The model under review builds one solid part; all positions refer to its coordinate system, in mm. Face numbers are marked on the shaded views. A direction names the side the tool comes from. Round coordinates to 2 decimals unless told otherwise and drop trailing zeros. Order: outer loops, then holes, each group sorted by start corner. A loop starts at its lowest first (then second) coordinate and runs counter-clockwise, first axis right, second up.
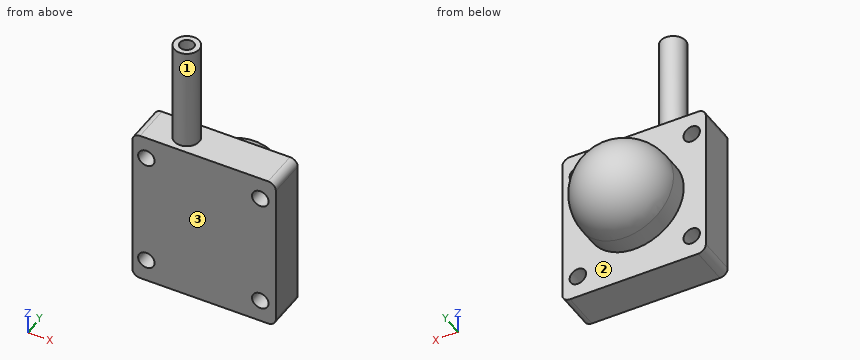
```python
from build123d import *

# Parameters (mm, degrees)
SKETCH1_W           = 27.860395724
SKETCH1_H           = 30.792543072
SKETCH1_R           = 1.6
BOSS_EXTRUDE1_DEPTH = 7.5
SKETCH2_R           = 9.5
BOSS_EXTRUDE2_DEPTH = 3.5
REVOLVE3_ANGLE      = 180
FILLET1_R           = 1.5
SKETCH4_R           = 2.416047387
SKETCH4_R_2         = 1.358434459
BOSS_EXTRUDE3_DEPTH = 20


with BuildPart() as part:
    # Sketch1 → Boss-Extrude1 (new body)
    with BuildSketch(Plane(origin=(0, 0, 0), x_dir=(1, 0, 0), z_dir=(0, 1, 0))):
        with Locations((0.138729437, 0)):
            Rectangle(SKETCH1_W, SKETCH1_H)
        with Locations(Location((-11.05, 11.05, 0), (0, 0, 270))):
            Circle(SKETCH1_R, mode=Mode.SUBTRACT)
        with Locations(Location((11.05, 11.05, 0), (0, 0, 270))):
            Circle(SKETCH1_R, mode=Mode.SUBTRACT)
        with Locations(Location((-11.05, -11.05, 0), (0, 0, 90))):
            Circle(SKETCH1_R, mode=Mode.SUBTRACT)
        with Locations(Location((11.05, -11.05, 0), (0, 0, 90))):
            Circle(SKETCH1_R, mode=Mode.SUBTRACT)
    extrude(amount=BOSS_EXTRUDE1_DEPTH)

    # Sketch2 → Boss-Extrude2 (add)
    with BuildSketch(Plane(origin=(0, 7.5, 0), x_dir=(1, 0, 0), z_dir=(0, 1, 0))):
        with Locations(Location((0, 0, 0), (0, 0, 270))):
            Circle(SKETCH2_R)
    extrude(amount=BOSS_EXTRUDE2_DEPTH)

    # Sketch3 → Revolve3 (revolve)
    with BuildSketch(Plane(origin=(0, 11, 0), x_dir=(1, 0, 0), z_dir=(0, 1, 0))):
        with BuildLine():
            Line((-9.5, 0), (9.5, 0))
            ThreePointArc((9.5, 0), (0, 9.5), (-9.5, 0))
        make_face()
    revolve(axis=Axis((-9.5, 11, 0), (1, 0, 0)), revolution_arc=REVOLVE3_ANGLE)

    # Fillet1
    fillet1_edges = [part.edges().sort_by_distance(p)[0] for p in [
        (-13.791468425, 3.75, -15.396271536),
        (14.068927299, 3.75, -15.396271536),
        (14.068927299, 3.75, 15.396271536),
        (-13.791468425, 3.75, 15.396271536),
    ]]
    fillet(fillet1_edges, radius=FILLET1_R)

    # Sketch4 → Boss-Extrude3 (add)
    with BuildSketch(Plane.XY.offset(15.396271536)):
        with Locations(Location((-5.220214875, 3.559374136, 0), (0, 0, 180))):
            Circle(SKETCH4_R)
        with Locations((-5.220214875, 3.559374136)):
            Circle(SKETCH4_R_2, mode=Mode.SUBTRACT)
    extrude(amount=BOSS_EXTRUDE3_DEPTH)


solid = part.part
```
(1) Insertion check: pin 1 (14 mm diameter, centred on x = 2.5, z = -5, fed in from +Y); pin 2 (1.5 mm diameter, centred on x = 0, z = 2, fed in from +Y); pin 3 (3 mm diameter, centred on y = 3, z = 16, fed in from -X). Each pin has a flat end and moves straight along its axis. Give the tip position at first contact, or say it passes through.
Data:
pin 1: stops at y = 20.5
pin 2: stops at y = 20.42
pin 3: stops at x = -13.66
(2) Consider section D-D (x = 0). Write out the cut boundary in (y, z), and give its area (3 significant figures).
Data:
outline: (0, -15.4) - (7.5, -15.4) - (7.5, -9.5) - (11, -9.5) arc R9.5 ccw to (11, 9.5) - (7.5, 9.5) - (7.5, 15.4) - (0, 15.4) - close
area: 439 mm2
(3) Consider section C-C (y = 4.25). Write out the cut boundary in (x, z).
Data:
outline: (-13.79, -13.9) arc R1.5 ccw to (-12.29, -15.4) - (12.57, -15.4) arc R1.5 ccw to (14.07, -13.9) - (14.07, 13.9) arc R1.5 ccw to (12.57, 15.4) - (-2.9, 15.4) - (-2.9, 35.4) - (-4.05, 35.4) - (-4.05, 15.4) - (-6.39, 15.4) - (-6.39, 35.4) - (-7.54, 35.4) - (-7.54, 15.4) - (-12.29, 15.4) arc R1.5 ccw to (-13.79, 13.9) - close; hole circle Ø3.2 at (-11.05, -11.05); hole circle Ø3.2 at (-11.05, 11.05); hole circle Ø3.2 at (11.05, -11.05); hole circle Ø3.2 at (11.05, 11.05)
(4) Consider section A-A (z = 11.05). Write out the cut boundary in (x, y).
Data:
outline: (-13.79, 0) - (-12.65, 0) - (-12.65, 7.5) - (-13.79, 7.5) - close; (-9.45, 0) - (9.45, 0) - (9.45, 7.5) - (-9.45, 7.5) - close; (12.65, 0) - (14.07, 0) - (14.07, 7.5) - (12.65, 7.5) - close
(5) Consider section B-B (x = -11.05). Write out the cut boundary in (y, z), and give its area (3 significant figures).
Data:
outline: (0, -15.4) - (7.5, -15.4) - (7.5, -12.65) - (0, -12.65) - close; (0, -9.45) - (7.5, -9.45) - (7.5, 9.45) - (0, 9.45) - close; (0, 12.65) - (7.5, 12.65) - (7.5, 15.4) - (0, 15.4) - close
area: 183 mm2
(6) To check wall thickness, follow probe 1 along X at (y, z) = (5.25, 11.05); probe 2 along Z at (x, y) = (-12, 4.75); probe 3 along Z at (x, y) = (0.25, 8.75). State the ranges of each line that lie inside material, in increasing order.
Data:
probe 1: x = -13.79 to -12.65, -9.45 to 9.45, 12.65 to 14.07
probe 2: z = -15.4 to -12.34, -9.76 to 9.76, 12.34 to 15.4
probe 3: z = -9.5 to 9.5
(7) For the marked faces 1, 2 and 3, list the 3-axis set-ups (+Z, -Z, +X, -X, +Y, -Y) from which the entire face can be reached by the end or side of a thin tool; tool diameter is ignored.
Data:
face 1: +Z
face 2: +Y
face 3: +Z, -Z, +X, -X, -Y
